from build123d import *

# Parameters (mm, degrees)
SKETCH_1_W          = 50
SKETCH_1_H          = 248
EXTRUDE_1_DEPTH     = 25
SKETCH_2_R          = 10.5
CUT_EXTRUDE_1_DEPTH = 26
CHAMFER_1_SIZE      = 6
CHAMFER_1_SIZE2     = 10.392304845
CHAMFER_2_SIZE      = 6
CHAMFER_2_SIZE2     = 10.392304845
CHAMFER_3_SIZE      = 1


with BuildPart() as part:
    # Эскиз1 → Бобышка-Вытянуть1 (new body)
    with BuildSketch(Plane.XY):
        with Locations((25, 124)):
            Rectangle(SKETCH_1_W, SKETCH_1_H)
    extrude(amount=EXTRUDE_1_DEPTH)

    # Эскиз2 → Вырез-Вытянуть1 (cut, through all)
    with BuildSketch(Plane.XY.offset(25)):
        with Locations((25, 23)):
            Circle(SKETCH_2_R)
        with Locations((25, 73)):
            Circle(SKETCH_2_R)
        with Locations((25, 123)):
            Circle(SKETCH_2_R)
        with Locations((25, 173)):
            Circle(SKETCH_2_R)
        with Locations((25, 223)):
            Circle(SKETCH_2_R)
    extrude(amount=-CUT_EXTRUDE_1_DEPTH, mode=Mode.SUBTRACT)

    # Фаска1
    chamfer_1_edges = [part.edges().sort_by_distance(p)[0] for p in [
        (25, 0, 0),
    ]]
    chamfer_1_side = [part.faces().sort_by_distance(p)[0] for p in [
        (25, 2.529901184, 0),
    ]]
    chamfer(chamfer_1_edges, length=CHAMFER_1_SIZE, length2=CHAMFER_1_SIZE2, reference=chamfer_1_side[0])

    # Фаска2
    chamfer_2_edges = [part.edges().sort_by_distance(p)[0] for p in [
        (25, 0, 25),
    ]]
    chamfer_2_side = [part.faces().sort_by_distance(p)[0] for p in [
        (25, 2.529901184, 25),
    ]]
    chamfer(chamfer_2_edges, length=CHAMFER_2_SIZE, length2=CHAMFER_2_SIZE2, reference=chamfer_2_side[0])

    # Фаска3
    chamfer_3_edges = [part.edges().sort_by_distance(p)[0] for p in [
        (14.5, 23, 0),
        (14.5, 23, 25),
        (14.5, 73, 0),
        (14.5, 73, 25),
        (14.5, 123, 0),
        (14.5, 123, 25),
        (14.5, 173, 0),
        (14.5, 173, 25),
        (14.5, 223, 0),
        (14.5, 223, 25),
    ]]
    chamfer(chamfer_3_edges, length=CHAMFER_3_SIZE)


solid = part.part
Input: part model. Units: mm. Frame: model coordinates. Coordinates: 2 decimals unless noted, no trailing zeros. Order: outer loops, then holes, each group sorted by start corner. A loop starts at its lowest first (then second) coordinate and runs counter-clockwise, first axis right, second up. Notation, with made-up numbers: M 87.25,-40 L 129.25,-40 A17 cw 129.25,-34 Z; hole C 14.25,9.5 d6. An arc over 180 degrees is marked long. Answer in a Markdown table with one row per item.
(1) Material intervals for line 1 (Y direction, x = 25, z = 10.75); line 2 (Y direction, x = 18.5, z = 16.75); line 3 (X direction, y = 124, z = 9.25), sorted ascending. Write a range as [from, to].
Numbers:
| item | result |
|---|---|
| line 1 | y = [0, 12.5], [33.5, 62.5], [83.5, 112.5], [133.5, 162.5], [183.5, 212.5], [233.5, 248] |
| line 2 | y = [1.24, 14.75], [31.25, 64.75], [81.25, 114.75], [131.25, 164.75], [181.25, 214.75], [231.25, 248] |
| line 3 | x = [0, 14.55], [35.45, 50] |
(2) Draft query along X for faces 1 (the flat face through (24.65, 2.958, 5.269)), 2 (the cylindrical face through (22.72, 112.75, 12.66)), 3 (the flat face through (0, 122, 12)). Return one class per face: pulls with the +X half, pulls with the -X half, needs draft (parallel to the pull), parting line crosses it, or undercut.
Numbers:
| item | result |
|---|---|
| face 1 | needs draft |
| face 2 | undercut |
| face 3 | pulls with the -X half |
(3) Section query A-A, the plane y = 23. Output: boundary loops of the cut face in (x, z), plus the area to 3 significant figures.
Numbers:
| item | result |
|---|---|
| outline | M 0,0 L 13.5,0 L 14.5,1 L 14.5,24 L 13.5,25 L 0,25 Z; M 35.5,1 L 36.5,0 L 50,0 L 50,25 L 36.5,25 L 35.5,24 Z |
| area | 723 mm^2 |
(4) Section query D-D, the plane z = 18.25. Output: boundary loops of the cut face in (x, y), plus the area to 3 significant figures.
Numbers:
| item | result |
|---|---|
| outline | M 0,2.1 L 50,2.1 L 50,248 L 0,248 Z; hole C 25,23 d21; hole C 25,73 d21; hole C 25,123 d21; hole C 25,173 d21; hole C 25,223 d21 |
| area | 10,600 mm^2 |
(5) Contact query for flat-ended pins moving along their axis: pin 1 Ø12 at (x, y) = (14.5, 138.5) entering from -Z; pin 2 Ø8 at (x, z) = (32.5, 21) entering from -Y. Output: stop coordinate, or through.
Numbers:
| item | result |
|---|---|
| pin 1 | stops at z = 0 |
| pin 2 | stops at y = 1.38 |
(6) Section query B-B, the plane z = 5.5. Output: boundary loops of the cut face in (x, y).
Numbers:
| item | result |
|---|---|
| outline | M 0,2.82 L 50,2.82 L 50,248 L 0,248 Z; hole C 25,23 d21; hole C 25,73 d21; hole C 25,123 d21; hole C 25,173 d21; hole C 25,223 d21 |
(7) Section query C-C, the plane x = 25. Give the number of separate pieces and of enclosed holes in the cut face, plus the area to 3 significant figures.
Numbers:
| item | result |
|---|---|
| separate pieces | 6 |
| enclosed holes | 0 |
| area | 3,500 mm^2 |
